```python
from build123d import *

# Parameters (mm, degrees)
BOSS_EXTRUDE1_DEPTH       = 1.5875
F_6_CLEARANCE_HOLE1_D     = 3.7973
F_6_CLEARANCE_HOLE2_D     = 3.7973
F_6_CLEARANCE_HOLE2_DEPTH = 25.4
F_6_CLEARANCE_HOLE2_TIP   = 1.140824014
F_6_CLEARANCE_HOLE3_D     = 3.7973
F_6_CLEARANCE_HOLE3_DEPTH = 25.4
F_6_CLEARANCE_HOLE3_TIP   = 1.140824014


with BuildPart() as part:
    # Sketch11 → Boss-Extrude1 (new body)
    with BuildSketch(Plane(origin=(0, 0, 0), x_dir=(1, 0, 0), z_dir=(0, 1, 0))):
        with BuildLine():
            Line((177.8, 38.1), (76.2, 38.1))
            add(Edge.make_bspline(
                [(76.2, 38.1), (-76.2, 38.1), (-76.2, -38.1), (76.2, -38.1)],
                knots=[0, 0, 0, 0, 1, 1, 1, 1], degree=3, weights=[1, 0.333333333, 0.333333333, 1]))
            Line((76.2, -38.1), (177.8, -38.1))
            add(Edge.make_bspline(
                [(177.8, -38.1), (431.8, -38.1), (431.8, 38.1), (177.8, 38.1)],
                knots=[0, 0, 0, 0, 1, 1, 1, 1], degree=3, weights=[1, 0.333333333, 0.333333333, 1]))
        make_face()
    extrude(amount=BOSS_EXTRUDE1_DEPTH)

    # #6 Clearance Hole1 (through all)
    with Locations(Plane(origin=(0, 0, 0), x_dir=(-1, 0, 0), z_dir=(0, -1, 0))):
        with Locations((-104.775, -28.575), (-149.225, -28.575), (-149.225, 28.575), (-104.775, 28.575)):
            Hole(F_6_CLEARANCE_HOLE1_D / 2)

    # #6 Clearance Hole2
    with Locations(Plane(origin=(0, 0, 0), x_dir=(-1, 0, 0), z_dir=(0, -1, 0))):
        with Locations((-19.05, 0)):
            Hole(F_6_CLEARANCE_HOLE2_D / 2, depth=F_6_CLEARANCE_HOLE2_DEPTH)
            with Locations((0, 0, -(F_6_CLEARANCE_HOLE2_DEPTH + F_6_CLEARANCE_HOLE2_TIP / 2))):  # 118° drill point
                Cone(0, F_6_CLEARANCE_HOLE2_D / 2, F_6_CLEARANCE_HOLE2_TIP, mode=Mode.SUBTRACT)

    # #6 Clearance Hole3
    with Locations(Plane(origin=(0, 0, 0), x_dir=(-1, 0, 0), z_dir=(0, -1, 0))):
        with Locations((-276.225, 0)):
            Hole(F_6_CLEARANCE_HOLE3_D / 2, depth=F_6_CLEARANCE_HOLE3_DEPTH)
            with Locations((0, 0, -(F_6_CLEARANCE_HOLE3_DEPTH + F_6_CLEARANCE_HOLE3_TIP / 2))):  # 118° drill point
                Cone(0, F_6_CLEARANCE_HOLE3_D / 2, F_6_CLEARANCE_HOLE3_TIP, mode=Mode.SUBTRACT)


solid = part.part
```
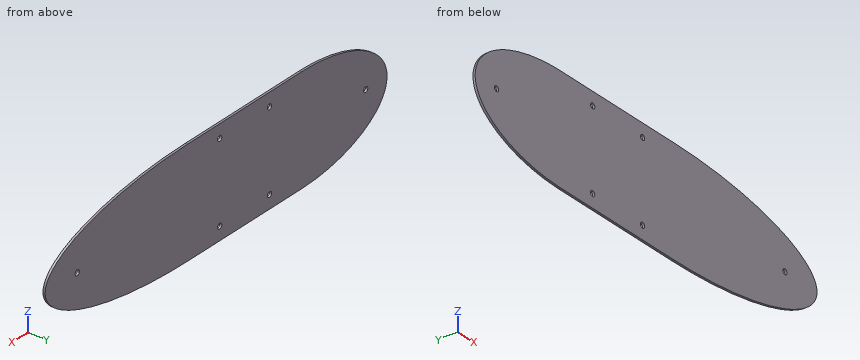
Work out the finished part from the listing and answer in its coordinate system (mm). Give positions to 0.01 mm unless a question says otherwise; leave off trailing zeros. Write each question's results on one line, items separated by ' | '.
1. This flat-tipped pin is pushed along its axis until it touches: pin 1 Ø2.5 at (x, z) = (149.225, -28.575) entering from -Y. Where does it stop, or does it pass through?
Data:
pin 1: through
2. Find section A-A on y = 1.2. Give the number of separate pieces and of enclosed holes in the cut face, and give its area (3 significant figures).
Data:
separate pieces: 1 | enclosed holes: 6 | area: 19,800 mm^2
3. Straight lines are drawn through the part: L1, parallel to X at y = 0.7, z = -13.5; L2, parallel to Z at x = 204, y = 1.2; L3, parallel to X at y = 0.35, z = 16. For each, find the intervals that lie inside material, in ascending order.
Data:
L1: 4.94 to 296.56 | L2: -37.28 to 37.28 | L3: 7.04 to 293.06
